```python
from build123d import *

# Parameters (mm, degrees)
SKETCH1_R           = 2.65
BOSS_EXTRUDE1_DEPTH = 2
SKETCH2_R           = 1.43
BOSS_EXTRUDE2_DEPTH = 12.5
FILLET1_R           = 0.5
FILLET2_R           = 0.1
CUT_EXTRUDE1_DEPTH  = 0.5
CUT_EXTRUDE1_TAPER  = 1


with BuildPart() as part:
    # Sketch1 → Boss-Extrude1 (new body)
    with BuildSketch(Plane(origin=(0, 0, 0), x_dir=(1, 0, 0), z_dir=(0, 1, 0))):
        Circle(SKETCH1_R)
    extrude(amount=BOSS_EXTRUDE1_DEPTH)

    # Sketch2 → Boss-Extrude2 (add)
    with BuildSketch(Plane.XZ):
        Circle(SKETCH2_R)
    extrude(amount=BOSS_EXTRUDE2_DEPTH)

    # Fillet1
    fillet1_edges = [part.edges().sort_by_distance(p)[0] for p in [
        (-2.65, 2, 0),
    ]]
    fillet(fillet1_edges, radius=FILLET1_R)

    # Fillet2
    fillet2_edges = [part.edges().sort_by_distance(p)[0] for p in [
        (-2.65, 0, 0),
    ]]
    fillet(fillet2_edges, radius=FILLET2_R)

    # Sketch3 → Cut-Extrude1 (cut)
    with BuildSketch(Plane(origin=(0, 2, 0), x_dir=(1, 0, 0), z_dir=(0, 1, 0))):
        Polygon((0.296573117, 0.3), (0.296573117, 1.336133674), (-0.303426883, 1.336133674), (-0.303426883, 0.3), (-1.340662941, 0.3), (-1.340662941, -0.3), (-0.303426883, -0.3), (-0.303426883, -1.336133674), (0.296573117, -1.336133674), (0.296573117, -0.3), (1.340662941, -0.3), (1.340662941, 0.3), align=None)
    extrude(amount=-CUT_EXTRUDE1_DEPTH, taper=CUT_EXTRUDE1_TAPER, mode=Mode.SUBTRACT)


solid = part.part
```
Part model, mm, in its own coordinate system. A direction names the side the tool comes from. Round coordinates to 2 decimals unless told otherwise and drop trailing zeros. Order: outer loops, then holes, each group sorted by start corner. A loop starts at its lowest first (then second) coordinate and runs counter-clockwise, first axis right, second up. Notation, with made-up numbers: M 75.25,29 L 109.25,29 A23 cw 109.25,53 Z; hole C 60,50 d8. An arc over 180 degrees is marked long. Put each result on its own line as item: value. Start each with the question number.
1. Slice it at A-A on y = -1.75. List the corners of the cut face in (x, z).
2. Tool access for faces 1 (the face through (0, 0, 2)), 2 (the face through (0, -12.5, 0)): list every direction of +Z, -Z, +X, -X, +Y, -Y with a clear straight run to the whole face (end or side of a thin tool).
3. Drill centre lines: probe 1 along Y at (x, z) = (-1.65, 0.15); probe 2 along Z at (x, y) = (0.05, -4.5); probe 3 along Y at (x, z) = (0.3, 0.2). Where is each one in solid material? Low to high. Write a range as [from, to].
4. Two-plate mould, pull along Z, no slides. Class faces 3 (the face through (2.45, 0.79, 1.01)), 4 (the face through (0.45, 2, 0.45)), 5 (the face through (0, 1.5, 0)): +Z half, -Z half, draft (parallel to the pull), parting line (faces both ways), or undercut.
5. Drop flat-ended pins along their axis: pin 1 (3 mm diameter, centred on x = 0.5, y = -7, fed in from -Z); pin 2 (1 mm diameter, centred on x = 1, y = 0, fed in from -Z); pin 3 (1 mm diameter, centred on x = -0.5, y = -9.5, fed in from +Z). Give the stop position or say it passes through.
Findings:
1. outline: C 0,0 d2.86
2. face 1: -Y
2. face 2: +Z, -Z, +X, -X, -Y
3. probe 1: [0, 2]
3. probe 2: [-1.43, 1.43]
3. probe 3: [-12.5, 1.5]
4. face 3: parting line
4. face 4: draft
4. face 5: undercut
5. pin 1: z = -1.43
5. pin 2: z = -2.6
5. pin 3: z = 1.43
